Input: part model. Units: mm. Frame: model coordinates. Face numbers are marked on the shaded views. Give positions to 0.01 mm unless a question says otherwise; leave off trailing zeros. Loops run counter-clockwise (first coordinate to the right, second up) from the corner with the lowest first, then second, coordinate; pieces in that order, holes last. Notation, with made-up numbers: (-15.5, -20.75) -> (31.5, -20.75) arc R11 ccw to (31.5, -7.75) -> close; hole circle Ø1 at (65.25, 71). An arc over 180 degrees is marked (long way). Answer as a JSON object with one key per item and string values. Group by question number.
```python
from build123d import *

# Parameters (mm, degrees)
F0_W     = 60
F0_H     = 105
F0_R     = 7.5
F1_DEPTH = 20
F2_DEPTH = 25
F3_R     = 2.5


with BuildPart() as f1:
    # F0 (on Top) → F1 (new body)
    with BuildSketch(Plane.XY):
        Rectangle(F0_W, F0_H)
        with Locations((0, -25)):
            Circle(F0_R, mode=Mode.SUBTRACT)
        Circle(F0_R, mode=Mode.SUBTRACT)
        with Locations((0, 25)):
            Circle(F0_R, mode=Mode.SUBTRACT)
    extrude(amount=F1_DEPTH)

    # F0 (on Top) → F2 (join)
    with BuildSketch(Plane.XY):
        Rectangle(F0_W, F0_H)
        with Locations((0, -25)):
            Circle(F0_R, mode=Mode.SUBTRACT)
        Circle(F0_R, mode=Mode.SUBTRACT)
        with Locations((0, 25)):
            Circle(F0_R, mode=Mode.SUBTRACT)
    extrude(amount=F2_DEPTH)

    # F3
    f3_edges = [f1.edges().sort_by_distance(p)[0] for p in [
        (-30, 0, 25),
        (0, 52.5, 25),
        (30, 0, 25),
        (0, -52.5, 25),
        (-30, 0, 0),
        (0, 52.5, 0),
        (30, 0, 0),
        (0, -52.5, 0),
    ]]
    fillet(f3_edges, radius=F3_R)


solid = f1.part
```
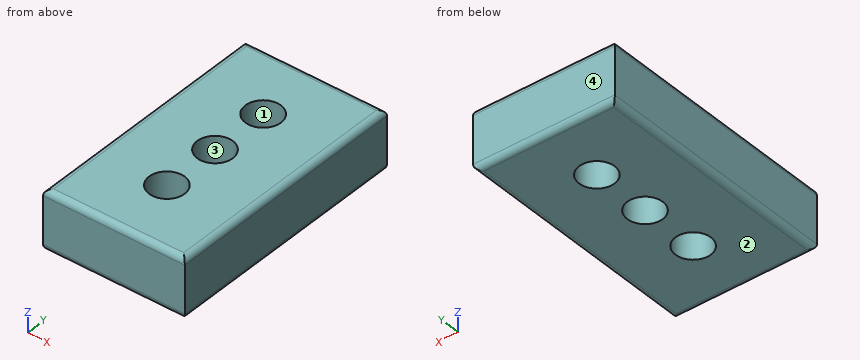
Q1. Section B-B on y = -25. Return the cut outline in (x, z).
Q2. Section D-D on y = 30. Return the cut outline in (x, z).
Q3. Pin query (flat end, axial travel): pin 1 Ø4 at (x, y) = (0.5, 29) entering from -Z. Return the tip coordinate at first contact, or that it passes through.
Q4. Pull-direction query (Y, two-part tool) for the marked faces 1, 2, 3 and 4; classes: +Y half, -Y half, draft (parallel to the pull), parting line (faces both ways), or undercut.
Q5. Section C-C on z = 8.5. Return the cut outline in (x, y), then the cut area to 3 significant figures.
Q6. Section A-A on x = 0. Return the cut outline in (y, z), then the cut area to 3 significant figures.
Q7. Ray query, probe 1 along Y at (x, z) = (0, 12.5); probe 2 along Y at (x, z) = (2, 21.25); probe 3 along X at (y, z) = (-4.5, 21.5). Return the intervals inside material, ascending.
Numbers:
{
 "1": {"outline": "(-30, 2.5) arc R2.5 ccw to (-27.5, 0) -> (-7.5, 0) -> (-7.5, 25) -> (-27.5, 25) arc R2.5 ccw to (-30, 22.5) -> close; (7.5, 0) -> (27.5, 0) arc R2.5 ccw to (30, 2.5) -> (30, 22.5) arc R2.5 ccw to (27.5, 25) -> (7.5, 25) -> close"},
 "2": {"outline": "(-30, 2.5) arc R2.5 ccw to (-27.5, 0) -> (-5.59, 0) -> (-5.59, 25) -> (-27.5, 25) arc R2.5 ccw to (-30, 22.5) -> close; (5.59, 0) -> (27.5, 0) arc R2.5 ccw to (30, 2.5) -> (30, 22.5) arc R2.5 ccw to (27.5, 25) -> (5.59, 25) -> close"},
 "3": {"pin 1": "passes through"},
 "4": {"face 1": "undercut", "face 2": "draft", "face 3": "undercut", "face 4": "+Y half"},
 "5": {"outline": "(-30, -52.5) -> (30, -52.5) -> (30, 52.5) -> (-30, 52.5) -> close; hole circle Ø15 at (0, -25); hole circle Ø15 at (0, 0); hole circle Ø15 at (0, 25)", "area": "5,770 mm²"},
 "6": {"outline": "(-52.5, 2.5) arc R2.5 ccw to (-50, 0) -> (-32.5, 0) -> (-32.5, 25) -> (-50, 25) arc R2.5 ccw to (-52.5, 22.5) -> close; (-17.5, 0) -> (-7.5, 0) -> (-7.5, 25) -> (-17.5, 25) -> close; (7.5, 0) -> (17.5, 0) -> (17.5, 25) -> (7.5, 25) -> close; (32.5, 0) -> (50, 0) arc R2.5 ccw to (52.5, 2.5) -> (52.5, 22.5) arc R2.5 ccw to (50, 25) -> (32.5, 25) -> close", "area": "1,490 mm²"},
 "7": {"probe 1": "y = -52.5 to -32.5, -17.5 to -7.5, 7.5 to 17.5, 32.5 to 52.5", "probe 2": "y = -52.5 to -32.23, -17.77 to -7.23, 7.23 to 17.77, 32.23 to 52.5", "probe 3": "x = -30 to -6, 6 to 30"}
}
